The listing builds one solid part. Answer for the finished solid, in the listing's coordinates (mm). A direction names the side the tool comes from. Give positions to 0.01 mm unless a question says otherwise; leave off trailing zeros. Answer in a Markdown table with one row per item.
from build123d import *

# Parameters (mm, degrees)
SKETCH1_W                                  = 95.25
SKETCH1_H                                  = 44.45
BOSS_EXTRUDE1_DEPTH                        = 4.75
CUT_EXTRUDE1_DEPTH                         = 1.84
CUT_EXTRUDE2_DEPTH                         = 2.38
SKETCH4_R                                  = 1.714999999
CUT_EXTRUDE3_DEPTH                         = 53.769818552
SKETCH5_R                                  = 3.05
CUT_EXTRUDE4_DEPTH                         = 2.38
MIRROR1_AT_THE_SECOND_PLANE_COPY_1_SKETC_R = 1.714999999
MIRROR1_AT_THE_SECOND_PLANE_COPY_1_DEPTH   = 53.769818552
MIRROR1_AT_THE_SECOND_PLANE_COPY_2_SKETC_R = 3.05
MIRROR1_AT_THE_SECOND_PLANE_COPY_2_DEPTH   = 2.38
FILLET1_R                                  = 1.5875


with BuildPart() as part:
    # Sketch1 → Boss-Extrude1 (new body)
    with BuildSketch(Plane.XY):
        Rectangle(SKETCH1_W, SKETCH1_H)
    extrude(amount=BOSS_EXTRUDE1_DEPTH)

    # Sketch2 → Cut-Extrude1 (cut)
    with BuildSketch(Plane.XY.offset(4.75)):
        with BuildLine():
            ThreePointArc((-46.165, 19.1775), (-45.700032015, 20.300032015), (-44.5775, 20.765))
            Line((-44.5775, 20.765), (44.5775, 20.765))
            ThreePointArc((44.5775, 20.765), (45.700032015, 20.300032015), (46.165, 19.1775))
            Line((46.165, 19.1775), (46.165, -19.1775))
            ThreePointArc((46.165, -19.1775), (45.700032015, -20.300032015), (44.5775, -20.765))
            Line((44.5775, -20.765), (-44.5775, -20.765))
            ThreePointArc((-44.5775, -20.765), (-45.700032015, -20.300032015), (-46.165, -19.1775))
            Line((-46.165, -19.1775), (-46.165, 19.1775))
        make_face()
        with BuildLine():
            Line((-44.195, -17.2075), (-44.195, 17.2075))
            ThreePointArc((-44.195, 17.2075), (-43.730032015, 18.330032015), (-42.6075, 18.795))
            Line((-42.6075, 18.795), (42.6075, 18.795))
            ThreePointArc((42.6075, 18.795), (43.730032015, 18.330032015), (44.195, 17.2075))
            Line((44.195, 17.2075), (44.195, -17.2075))
            ThreePointArc((44.195, -17.2075), (43.730032015, -18.330032015), (42.6075, -18.795))
            Line((42.6075, -18.795), (-42.6075, -18.795))
            ThreePointArc((-42.6075, -18.795), (-43.730032015, -18.330032015), (-44.195, -17.2075))
        make_face(mode=Mode.SUBTRACT)
    extrude(amount=-CUT_EXTRUDE1_DEPTH, mode=Mode.SUBTRACT)

    # Sketch3 → Cut-Extrude2 (cut)
    with BuildSketch(Plane.XY.offset(4.75)):
        with BuildLine():
            Line((-36.257500002, 12.445), (36.257500002, 12.445))
            ThreePointArc((36.257500002, 12.445), (37.380032017, 11.980032015), (37.845000002, 10.8575))
            Line((37.845000002, 10.8575), (37.845000002, -10.8575))
            ThreePointArc((37.845000002, -10.8575), (37.380032017, -11.980032015), (36.257500002, -12.445))
            Line((36.257500002, -12.445), (-36.257500002, -12.445))
            ThreePointArc((-36.257500002, -12.445), (-37.380032017, -11.980032015), (-37.845000002, -10.8575))
            Line((-37.845000002, -10.8575), (-37.845000002, 10.8575))
            ThreePointArc((-37.845000002, 10.8575), (-37.380032017, 11.980032015), (-36.257500002, 12.445))
        make_face()
    extrude(amount=-CUT_EXTRUDE2_DEPTH, mode=Mode.SUBTRACT)

    # Sketch4 → Cut-Extrude3 (cut, through all)
    with BuildSketch(Plane.XY.offset(4.75)):
        with Locations((-41.275, 15.875)):
            Circle(SKETCH4_R)
    cut_extrude3 = extrude(amount=-CUT_EXTRUDE3_DEPTH, mode=Mode.SUBTRACT)

    # Sketch5 → Cut-Extrude4 (cut)
    with BuildSketch(Plane(origin=(0, 0, 0), x_dir=(-1, 0, 0), z_dir=(0, 0, -1))):
        with Locations((41.275, 15.875)):
            Circle(SKETCH5_R)
    cut_extrude4 = extrude(amount=-CUT_EXTRUDE4_DEPTH, mode=Mode.SUBTRACT)

    # Mirror1: Cut-Extrude3, Cut-Extrude4 across plane
    add(cut_extrude3.mirror(Plane(origin=(0, 0, 0), x_dir=(0, 0, 1), z_dir=(1, 0, 0))), mode=Mode.SUBTRACT)
    add(cut_extrude4.mirror(Plane(origin=(0, 0, 0), x_dir=(0, 0, 1), z_dir=(1, 0, 0))), mode=Mode.SUBTRACT)

    # Mirror1 at the second plane: Cut-Extrude3, Cut-Extrude4 across plane
    add(cut_extrude3.mirror(Plane.ZX), mode=Mode.SUBTRACT)
    add(cut_extrude4.mirror(Plane.ZX), mode=Mode.SUBTRACT)

    # Mirror1 at the second plane copy 1 sketc → Mirror1 at the second plane copy 1 (cut, through all)
    with BuildSketch(Plane(origin=(0, 0, 4.75), x_dir=(-1, 0, 0), z_dir=(0, 0, 1))):
        with Locations((-41.275, 15.875)):
            Circle(MIRROR1_AT_THE_SECOND_PLANE_COPY_1_SKETC_R)
    extrude(amount=-MIRROR1_AT_THE_SECOND_PLANE_COPY_1_DEPTH, mode=Mode.SUBTRACT)

    # Mirror1 at the second plane copy 2 sketc → Mirror1 at the second plane copy 2 (cut)
    with BuildSketch(Plane(origin=(0, 0, 0), x_dir=(1, 0, 0), z_dir=(0, 0, -1))):
        with Locations((41.275, 15.875)):
            Circle(MIRROR1_AT_THE_SECOND_PLANE_COPY_2_SKETC_R)
    extrude(amount=-MIRROR1_AT_THE_SECOND_PLANE_COPY_2_DEPTH, mode=Mode.SUBTRACT)

    # Fillet1
    fillet1_edges = [part.edges().sort_by_distance(p)[0] for p in [
        (0, -22.225, 0),
        (-47.625, 0, 0),
        (0, 22.225, 0),
        (47.625, 0, 0),
        (47.625, -22.225, 2.375),
        (-47.625, -22.225, 2.375),
        (-47.625, 22.225, 2.375),
        (47.625, 22.225, 2.375),
    ]]
    fillet(fillet1_edges, radius=FILLET1_R)


solid = part.part
Item 1: Consider line 1 (Y direction, x = -32, z = 3.95) (3 decimals); line 2 (X direction, y = -8, z = 3.4) (3 decimals); line 3 (Y direction, x = 29, z = 2.6) (3 decimals). Determine where each line is inside the solid, lowest interval first.
Answer block:
| item | result |
|---|---|
| line 1 | -22.225 to -20.765, -18.795 to -12.445, 12.445 to 18.795, 20.765 to 22.225 |
| line 2 | -47.625 to -46.165, -44.195 to -37.845, 37.845 to 44.195, 46.165 to 47.625 |
| line 3 | -22.225 to -12.445, 12.445 to 22.225 |
Item 2: Determine the mould class of faces 4 (the face through (47.15, 21.77, 3.19)), 5 (the face through (-43.74, 18.32, 3.84)), 6 (the face through (0.645, -21.772, 0.477)) for opening direction X: pulls with the +X half, pulls with the -X half, needs draft (parallel to the pull), parting line crosses it, or undercut.
Answer block:
| item | result |
|---|---|
| face 4 | pulls with the +X half |
| face 5 | undercut |
| face 6 | needs draft |
Item 3: Each of these flat-tipped pins is pushed along its axis until it touches: P1, Ø1, axis at y = -13, z = 1, coming from the -X side; P2, Ø12.5, axis at x = 9, y = -5.5, coming from the +Z side. Where does it stop, or does it pass through?
Answer block:
| item | result |
|---|---|
| P1 | x = -47.62 |
| P2 | z = 2.37 |
Item 4: Which of the six approach directions +Z, -Z, +X, -X, +Y, -Y give full straight-line access (tool end or side, diameter ignored) to faces 1 (the face through (47.625, 0, 3)), 2 (the face through (-1, 18.795, 4)), 3 (the face through (-44.184, -16.791, 1.173))?
Answer block:
| item | result |
|---|---|
| face 1 | +Z, -Z, +X, +Y, -Y |
| face 2 | +Z |
| face 3 | -Z |
